Part print with two shaded views. Sizes in mm from the minimum x, y, z corner. A direction names the side the tool comes from. Round coordinates to 2 decimals unless told otherwise and drop trailing zeros. Order: outer loops, then holes, each group sorted by start corner. A loop starts at its lowest first (then second) coordinate and runs counter-clockwise, first axis right, second up. Notation, with made-up numbers: M -28,40.5 L 25,40.5 A22 ccw 25,55.5 Z; hole C 15,6 d6. An arc over 180 degrees is marked long. One line per question, with ' | ' between items.
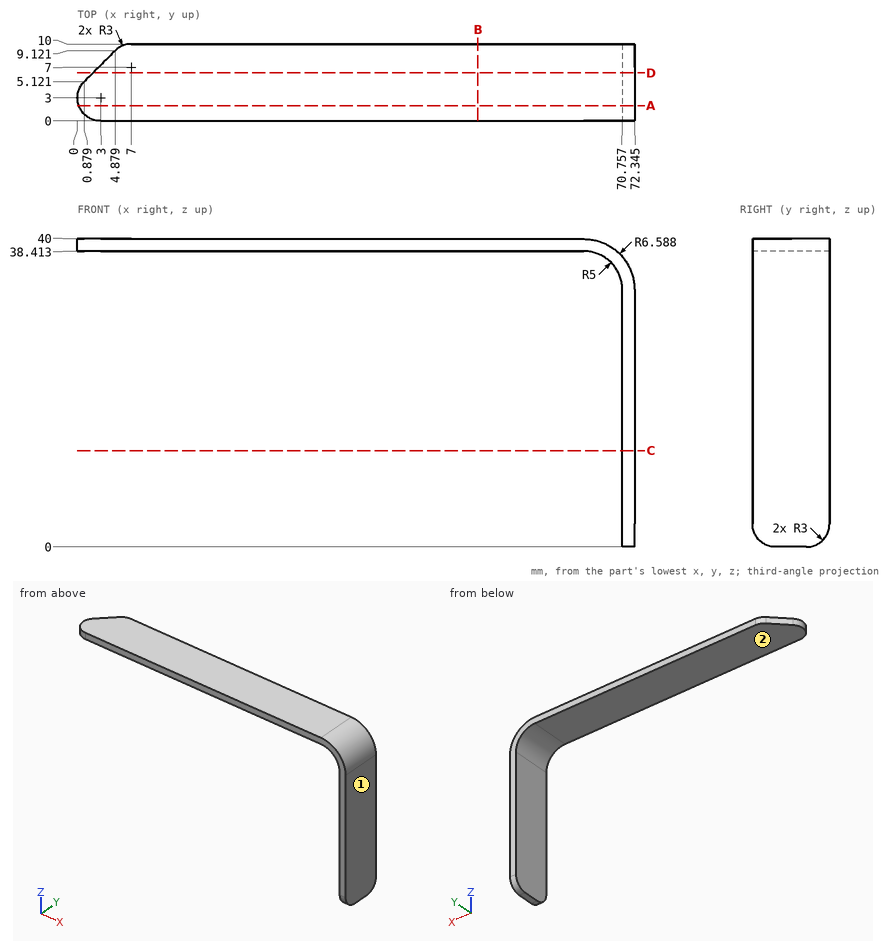
1) Saw through at B-B (x = 52). List the corners of the cut face in (y, z), plus the area to 3 significant figures.
The answers:
outline: M 0,38.41 L 10,38.41 L 10,40 L 0,40 Z | area: 15.9 mm²
2) Drop flat-ended pins along their axis: pin 1 (2 mm diameter, centred on x = 36, y = 1.5, fed in from -Z); pin 2 (3 mm diameter, centred on y = 7, z = 8.5, fed in from -X); pin 3 (12 mm diameter, centred on x = 53.5, z = 32.5, fed in from -Y). Give the stop position or say it passes through.
The answers:
pin 1: stops at z = 38.41 | pin 2: stops at x = 70.76 | pin 3: stops at y = 0
3) Probe line 1 (X direction, y = 5, z = 32) (1 decimal); line 2 (Z direction, x = 54, y = 9.25); line 3 (Z direction, x = 69.5, y = 9.75) (1 decimal). List the from-to ranges inside material, lowest first. Write a range as [from, to].
The answers:
line 1: x = [70.8, 72.3] | line 2: z = [38.41, 40] | line 3: z = [36.7, 38.8]
4) Saw through at D-D (y = 6.25). List the corners of the cut face in (x, z) (1 decimal).
The answers:
outline: M 2,38.4 L 65.8,38.4 A5 cw 70.8,33.4 L 70.8,0 L 72.3,0 L 72.3,33.4 A6.6 ccw 65.8,40 L 2,40 Z
5) Saw through at A-A (y = 2). List the corners of the cut face in (x, z) (1 decimal).
The answers:
outline: M 0.2,38.4 L 65.8,38.4 A5 cw 70.8,33.4 L 70.8,0.2 L 72.3,0.2 L 72.3,33.4 A6.6 ccw 65.8,40 L 0.2,40 Z
6) Which spindle directions (+Z, -Z, +X, -X, +Y, -Y) get a long thin tool onto all of the face, cutting with end or side? Do the marked faces 1 and 2. Say none if no direction does.
The answers:
face 1: +Z, -Z, +X, +Y, -Y | face 2: -Z, -X, +Y, -Y
7) Saw through at C-C (z = 12.5). List the corners of the cut face in (x, y) (1 decimal), plus the area to 3 significant figures.
The answers:
outline: M 70.8,0 L 72.3,0 L 72.3,10 L 70.8,10 Z | area: 15.9 mm²
